Check sheet for the modelled part. Datum: model origin and axes. Units: mm. A direction names the side the tool comes from. Coordinates: 2 decimals unless noted, no trailing zeros. Order: outer loops, then holes, each group sorted by start corner. A loop starts at its lowest first (then second) coordinate and runs counter-clockwise, first axis right, second up.
from build123d import *

# Parameters (mm, degrees)
SKETCH1_W           = 32
SKETCH1_H           = 87
SKETCH1_R           = 1.5
SKETCH1_W_2         = 10.5
SKETCH1_H_2         = 3.175
BOSS_EXTRUDE1_DEPTH = 3.175


with BuildPart() as part:
    # Sketch1 → Boss-Extrude1 (new body)
    with BuildSketch(Plane(origin=(0, 0, 0), x_dir=(1, 0, 0), z_dir=(0, 1, 0))):
        with Locations((16, 43.5)):
            Rectangle(SKETCH1_W, SKETCH1_H)
        with Locations((4.475, 72.525)):
            Circle(SKETCH1_R, mode=Mode.SUBTRACT)
        with Locations((27.525, 72.525)):
            Circle(SKETCH1_R, mode=Mode.SUBTRACT)
        with Locations((27.525, 14.475)):
            Circle(SKETCH1_R, mode=Mode.SUBTRACT)
        with Locations((4.475, 14.475)):
            Circle(SKETCH1_R, mode=Mode.SUBTRACT)
        with Locations((16, 6.0875)):
            Rectangle(SKETCH1_W_2, SKETCH1_H_2, mode=Mode.SUBTRACT)
        with Locations((16, 80.9125)):
            Rectangle(SKETCH1_W_2, SKETCH1_H_2, mode=Mode.SUBTRACT)
    extrude(amount=BOSS_EXTRUDE1_DEPTH)


solid = part.part
(1) Thickness scan on probe 1 along Z at (x, y) = (17.5, 2.25) (3 decimals); probe 2 along Z at (x, y) = (5, 0.35); probe 3 along X at (y, z) = (1.7, -72). Record the ranges inside material, lowest first.
Filled in:
probe 1: z = -87 to -82.5, -79.325 to -7.675, -4.5 to 0
probe 2: z = -87 to -73.93, -71.12 to -15.88, -13.07 to 0
probe 3: x = 0 to 3.07, 5.88 to 26.12, 28.93 to 32
(2) Cross-section at B-B (y = 0.55). Enter the section's corners in (x, z) (3 decimals).
Filled in:
outline: (0, -87) - (32, -87) - (32, 0) - (0, 0) - close; hole circle Ø3 at (4.475, -72.525); hole circle Ø3 at (4.475, -14.475); hole (10.75, -82.5) - (21.25, -82.5) - (21.25, -79.325) - (10.75, -79.325) - close; hole (10.75, -7.675) - (21.25, -7.675) - (21.25, -4.5) - (10.75, -4.5) - close; hole circle Ø3 at (27.525, -72.525); hole circle Ø3 at (27.525, -14.475)
(3) Cross-section at C-C (x = 4.5). Enter the section's corners in (y, z) (3 decimals), and give its area (3 significant figures).
Filled in:
outline: (0, -87) - (3.175, -87) - (3.175, -74.025) - (0, -74.025) - close; (0, -71.025) - (3.175, -71.025) - (3.175, -15.975) - (0, -15.975) - close; (0, -12.975) - (3.175, -12.975) - (3.175, 0) - (0, 0) - close
area: 257 mm2
(4) Cross-section at A-A (x = 15.5). Enter the section's corners in (y, z) (3 decimals).
Filled in:
outline: (0, -87) - (3.175, -87) - (3.175, -82.5) - (0, -82.5) - close; (0, -79.325) - (3.175, -79.325) - (3.175, -7.675) - (0, -7.675) - close; (0, -4.5) - (3.175, -4.5) - (3.175, 0) - (0, 0) - close
(5) Release check for a two-part mould opening along X. For faces 3 (the cylindrical face through (4.28, 1.565, -15.962)), 4 (the flat face through (0, 2, -43)), 5 (the flat face through (32, 2, -43)) record: +X half, -X half, draft (parallel to the pull), parting line (faces both ways), or undercut.
Filled in:
face 3: undercut
face 4: -X half
face 5: +X half
(6) Go/stop test with a flat-tipped pin: P1, Ø2.5, axis at x = 4.475, z = -72.525, coming from the +Y side. Record where the tip stops, or that it passes through.
Filled in:
P1: passes through
(7) Tool access check on faces 1 (the flat face through (16, 0, -44)), 2 (the flat face through (10.75, 2, -81)). Record the directions out of +Z, -Z, +X, -X, +Y, -Y that give a thin tool (end or side, any length) a straight path to the whole face; none if there is none.
Filled in:
face 1: +Z, -Z, +X, -X, -Y
face 2: +Y, -Y
